The drawing under review shows one solid part. Ordinate dimensions are in mm from its lowest x, y, z. Coordinates: 2 decimals unless noted, no trailing zeros. Loops run counter-clockwise (first coordinate to the right, second up) from the corner with the lowest first, then second, coordinate; pieces in that order, holes last. Notation, with made-up numbers: (23.5, 38) - (65.5, 38) arc R21 cw to (65.5, 59) - close; hole circle Ø8 at (83, 75.25). An arc over 180 degrees is marked (long way). Answer as a JSON object with one key per item and string values. Group by question number.
Item 1: We need section A-A (y = 31.75). Give the boundary of the cut face in (x, z), then the cut area to 3 significant figures.
Item 2: Clearance check with flat-ended pins moving along their axes: pin 1 (1.5 mm diameter, centred on y = 50, z = 1.5, fed in from +X); pin 2 (0.5 mm diameter, centred on x = 16, z = 2, fed in from +Y); pin 3 (1.1 mm diameter, centred on x = 0.5, z = 1, fed in from +Y). State where each tip first meets the part, or that it passes through.
Item 3: To check wall thickness, follow line 1 (Y direction, x = 11, z = 2.3); line 2 (X direction, y = 42, z = 0.3); line 3 (Y direction, x = 10.25, z = 2.55). State the ranges of each line that lie inside material, in increasing order.
Item 4: We need section C-C (z = 1.6). Give the boundary of the cut face in (x, y).
Item 5: We need section B-B (x = 11). Give the boundary of the cut face in (y, z), then the cut area to 3 significant figures.
Item 6: We need section D-D (y = 53.5). Give the boundary of the cut face in (x, z), then the cut area to 3 significant figures.
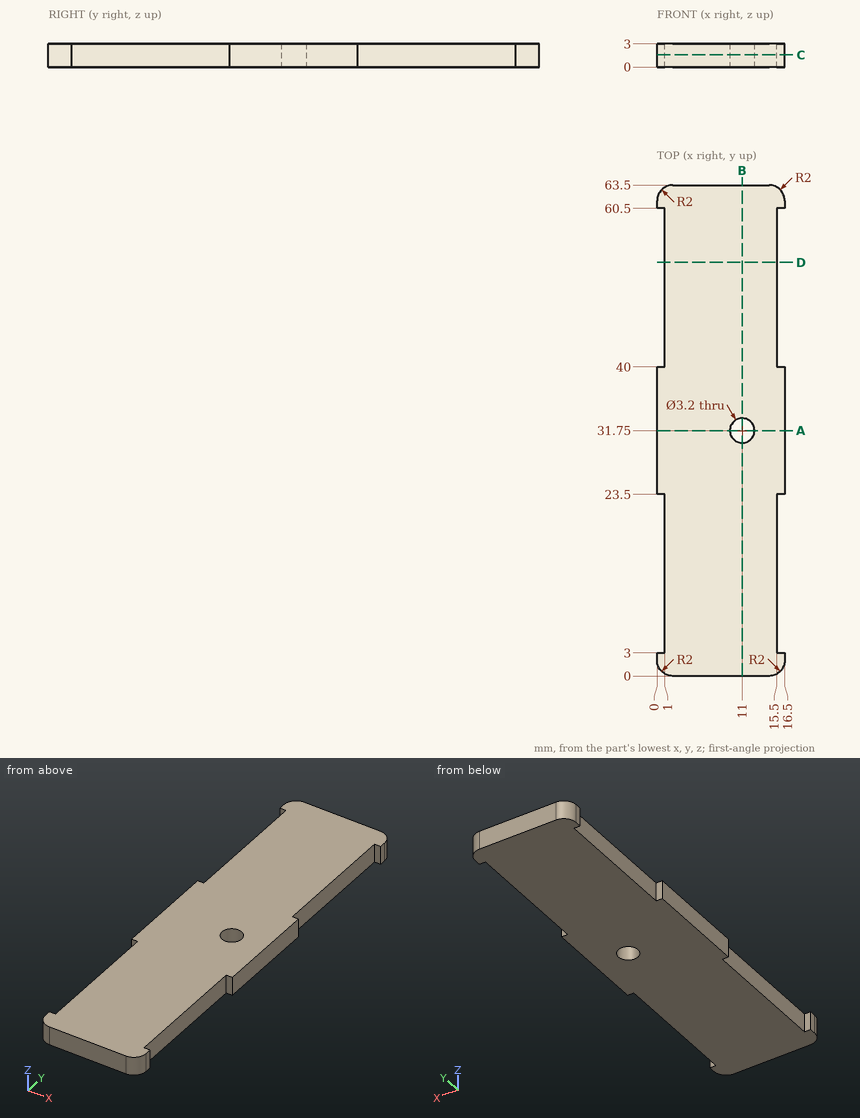
Check sheet entries:
{
 "1": {"outline": "(0, 0) - (9.4, 0) - (9.4, 3) - (0, 3) - close; (12.6, 0) - (16.5, 0) - (16.5, 3) - (12.6, 3) - close", "area": "39.9 mm2"},
 "2": {"pin 1": "stops at x = 15.5", "pin 2": "stops at y = 63.06", "pin 3": "stops at y = 63.26"},
 "3": {"line 1": "y = 0 to 30.15, 33.35 to 63.5", "line 2": "x = 1 to 15.5", "line 3": "y = 0 to 30.34, 33.16 to 63.5"},
 "4": {"outline": "(0, 2) arc R2 ccw to (2, 0) - (14.5, 0) arc R2 ccw to (16.5, 2) - (16.5, 3) - (15.5, 3) - (15.5, 23.5) - (16.5, 23.5) - (16.5, 40) - (15.5, 40) - (15.5, 60.5) - (16.5, 60.5) - (16.5, 61.5) arc R2 ccw to (14.5, 63.5) - (2, 63.5) arc R2 ccw to (0, 61.5) - (0, 60.5) - (1, 60.5) - (1, 40) - (0, 40) - (0, 23.5) - (1, 23.5) - (1, 3) - (0, 3) - close; hole circle Ø3.2 at (11, 31.75)"},
 "5": {"outline": "(0, 0) - (30.15, 0) - (30.15, 3) - (0, 3) - close; (33.35, 0) - (63.5, 0) - (63.5, 3) - (33.35, 3) - close", "area": "181 mm2"},
 "6": {"outline": "(1, 0) - (15.5, 0) - (15.5, 3) - (1, 3) - close", "area": "43.5 mm2"}
}
